Answer from the drawing. Dimensions are ordinates in mm from the lowest x, y and z of the part. A direction names the side the tool comes from. Round coordinates to 2 decimals unless told otherwise and drop trailing zeros. Order: outer loops, then holes, each group sorted by start corner. A loop starts at its lowest first (then second) coordinate and runs counter-clockwise, first axis right, second up. Notation, with made-up numbers: M 13,-15 L 71,-15 A34 ccw 71,17 Z; hole C 61,28 d2. An arc over 180 degrees is marked long. Write item = value, one per line. Start each with the question number.
(1) A cutting plane is placed at A-A, the plane y = 18.5. Determine the outline of the cut face in (x, z), and give its area (3 significant figures).
(2) A cutting plane is placed at D-D, the plane z = 51. Determine the outline of the cut face in (x, y).
(3) Which of the six approach directions +Z, -Z, +X, -X, +Y, -Y give full straight-line access (tool end or side, diameter ignored) to the marked faces 1 and 2?
(4) Straight lines are drawn through the part: probe 1 along Z at (x, y) = (15, 30.5) (1 decimal); probe 2 along Z at (x, y) = (15.5, 29.5) (1 decimal); probe 3 along Y at (x, z) = (18, 21.5) (1 decimal). For each, find the intervals that lie inside material, in ascending order. Write a range as from..to.
(5) Each of these flat-tipped pins is pushed along its axis until it touches: pin 1 (6 mm diameter, centred on y = 27, z = 121.5, fed in from +X); pin 2 (1.9 mm diameter, centred on y = 2, z = 94.5, fed in from +X); pin 3 (12 mm diameter, centred on y = 23.88, z = 125.41, fed in from +X); pin 4 (6.5 mm diameter, centred on x = 26.5, z = 99, fed in from -Y). Where does it stop, or does it pass through?
(6) A cutting plane is placed at C-C, the plane x = 7.5. Determine the outline of the cut face in (y, z) (1 decimal).
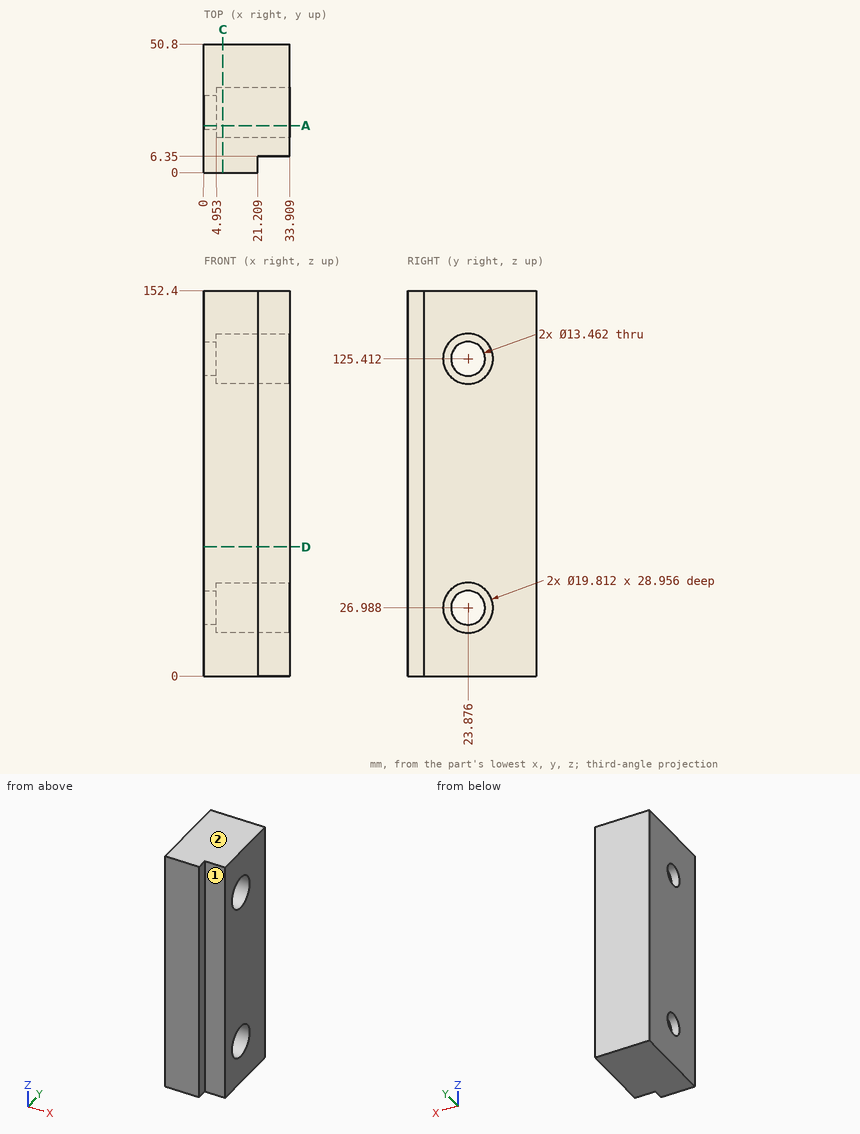
Reported:
q1.outline = M 0,0 L 33.91,0 L 33.91,18.67 L 4.95,18.67 L 4.95,22.94 L 0,22.94 Z; M 0,31.04 L 4.95,31.04 L 4.95,35.31 L 33.91,35.31 L 33.91,117.09 L 4.95,117.09 L 4.95,121.36 L 0,121.36 Z; M 0,129.46 L 4.95,129.46 L 4.95,133.73 L 33.91,133.73 L 33.91,152.4 L 0,152.4 Z
q1.area = 4,120 mm²
q2.outline = M 0,0 L 21.21,0 L 21.21,6.35 L 33.91,6.35 L 33.91,50.8 L 0,50.8 Z
q3.face_1 = +Z, -Z, +X, -Y
q3.face_2 = +Z, +X, -X, +Y, -Y
q4.probe_1 = 0..19.6, 34.4..118, 132.8..152.4
q4.probe_2 = 0..18.8, 35.1..117.3, 133.6..152.4
q4.probe_3 = 0..15.6, 32.1..50.8
q5.pin_1 = 4.95
q5.pin_2 = 21.21
q5.pin_3 = through
q5.pin_4 = 6.35
q6.outline = M 0,0 L 50.8,0 L 50.8,152.4 L 0,152.4 Z; hole C 23.9,27 d19.8; hole C 23.9,125.4 d19.8
